```python
from build123d import *

# Parameters (mm, degrees)
F0_W         = 40.5
F0_H         = 40.5
F2_W         = 32.47
F2_H         = 32.47
F4_W         = 38
F4_H         = 38
F5_W         = 30
F5_H         = 30
F7_W         = 40.5
F7_H         = 40.5
F7_R         = 1.5
F7_R_2       = 19
F8_DEPTH     = 2.3
F9_T3_DEPTH  = 22.3515662211
F9_T6_DEPTH  = 9.05
F9_T9_DEPTH  = 9.05
F9_T12_DEPTH = 22.3515662211
F9_T15_DEPTH = 22.3515662211
F9_T18_DEPTH = 9.05
F9_T21_DEPTH = 22.3515662211
F9_T24_DEPTH = 9.05
F9_T27_DEPTH = 36.3076821333


# Not quite as in the source:
# - a fillet or chamfer that OpenCascade refuses, or shapes differently, is made with other operations: its cross-section is extruded or revolved along the edge and cut away or added


with BuildPart() as f3:
    # F0 (on Top) → F3 section 0
    with BuildSketch(Plane.XY):
        Rectangle(F0_W, F0_H)
    # F2 (on offset) → F3 section 1
    with BuildSketch(Plane.XY.offset(15)):
        Rectangle(F2_W, F2_H)
    loft()

    # F4 (on face) → F6 section 0
    with BuildSketch(Plane.XY):
        Rectangle(F4_W, F4_H)
    # F5 (on face) → F6 section 1
    with BuildSketch(Plane.XY.offset(15)):
        Rectangle(F5_W, F5_H)
    loft(mode=Mode.SUBTRACT)

    # F7 (on face) → F8 (join)
    with BuildSketch(Plane.XY):
        Rectangle(F7_W, F7_H)
        with Locations((-15.9099025767, -15.9099025767)):
            Circle(F7_R, mode=Mode.SUBTRACT)
        with Locations((15.9099025767, -15.9099025767)):
            Circle(F7_R, mode=Mode.SUBTRACT)
        with Locations((-15.9099025767, 15.9099025767)):
            Circle(F7_R, mode=Mode.SUBTRACT)
        Circle(F7_R_2, mode=Mode.SUBTRACT)
        with Locations((15.9099025767, 15.9099025767)):
            Circle(F7_R, mode=Mode.SUBTRACT)
    extrude(amount=-F8_DEPTH)

    # F9: fillet of radius 1 on 9 edges, made by hand


with BuildPart() as f9_tool1:
    # F9_s2 → F9_t3 (new body)
    with BuildSketch(Plane(origin=(-3.5329799901, -3.5329799901, -13.1991780453), x_dir=(-0.7071067812, 0.7071067812, 0), z_dir=(0.2503317407, 0.2503317407, 0.9352368893))):
        with BuildLine():
            ThreePointArc((-0.6830609237, 26.1443262584), (0, 26.4139648585), (0.6830609237, 26.1443262584))
            Line((0.6830609237, 26.1443262584), (0, 26.783150032))
            Line((0, 26.783150032), (-0.6830609237, 26.1443262584))
        make_face()
    extrude(amount=F9_T3_DEPTH)


with BuildPart() as f9_tool4:
    # F9_s5 → F9_t6 (new body)
    with BuildSketch(Plane.XY.offset(4.25)):
        with BuildLine():
            ThreePointArc((-19.25, -20.25), (-19.9571067812, -19.9571067812), (-20.25, -19.25))
            Line((-20.25, -19.25), (-20.25, -20.25))
            Line((-20.25, -20.25), (-19.25, -20.25))
        make_face()
    extrude(amount=-F9_T6_DEPTH)


with BuildPart() as f9_tool7:
    # F9_s8 → F9_t9 (new body)
    with BuildSketch(Plane.XY.offset(4.25)):
        with BuildLine():
            ThreePointArc((-20.25, 19.25), (-19.9571067812, 19.9571067812), (-19.25, 20.25))
            Line((-19.25, 20.25), (-20.25, 20.25))
            Line((-20.25, 20.25), (-20.25, 19.25))
        make_face()
    extrude(amount=-F9_T9_DEPTH)


with BuildPart() as f9_tool10:
    # F9_s11 → F9_t12 (new body)
    with BuildSketch(Plane(origin=(-3.5329799901, 3.5329799901, -13.1991780453), x_dir=(0.7071067812, 0.7071067812, 0), z_dir=(0.2503317407, -0.2503317407, 0.9352368893))):
        with BuildLine():
            ThreePointArc((-0.6830609237, 26.1443262584), (0, 26.4139648585), (0.6830609237, 26.1443262584))
            Line((0.6830609237, 26.1443262584), (0, 26.783150032))
            Line((0, 26.783150032), (-0.6830609237, 26.1443262584))
        make_face()
    extrude(amount=F9_T12_DEPTH)


with BuildPart() as f9_tool13:
    # F9_s14 → F9_t15 (new body)
    with BuildSketch(Plane(origin=(3.5329799901, 3.5329799901, -13.1991780453), x_dir=(0.7071067812, -0.7071067812, 0), z_dir=(-0.2503317407, -0.2503317407, 0.9352368893))):
        with BuildLine():
            ThreePointArc((0.6830609237, 26.1443262584), (0, 26.4139648585), (-0.6830609237, 26.1443262584))
            Line((-0.6830609237, 26.1443262584), (0, 26.783150032))
            Line((0, 26.783150032), (0.6830609237, 26.1443262584))
        make_face()
    extrude(amount=F9_T15_DEPTH)


with BuildPart() as f9_tool16:
    # F9_s17 → F9_t18 (new body)
    with BuildSketch(Plane.XY.offset(4.25)):
        with BuildLine():
            ThreePointArc((20.25, 19.25), (19.9571067812, 19.9571067812), (19.25, 20.25))
            Line((19.25, 20.25), (20.25, 20.25))
            Line((20.25, 20.25), (20.25, 19.25))
        make_face()
    extrude(amount=-F9_T18_DEPTH)


with BuildPart() as f9_tool19:
    # F9_s20 → F9_t21 (new body)
    with BuildSketch(Plane(origin=(3.5329799901, -3.5329799901, -13.1991780453), x_dir=(-0.7071067812, -0.7071067812, 0), z_dir=(-0.2503317407, 0.2503317407, 0.9352368893))):
        with BuildLine():
            ThreePointArc((0.6830609237, 26.1443262584), (0, 26.4139648585), (-0.6830609237, 26.1443262584))
            Line((-0.6830609237, 26.1443262584), (0, 26.783150032))
            Line((0, 26.783150032), (0.6830609237, 26.1443262584))
        make_face()
    extrude(amount=F9_T21_DEPTH)


with BuildPart() as f9_tool22:
    # F9_s23 → F9_t24 (new body)
    with BuildSketch(Plane.XY.offset(4.25)):
        with BuildLine():
            ThreePointArc((19.25, -20.25), (19.9571067812, -19.9571067812), (20.25, -19.25))
            Line((20.25, -19.25), (20.25, -20.25))
            Line((20.25, -20.25), (19.25, -20.25))
        make_face()
    extrude(amount=-F9_T24_DEPTH)


with BuildPart() as f9_tool25:
    # F9_s26 → F9_t27 (new body)
    with BuildSketch(Plane.XZ.offset(-18.1538410667)):
        with BuildLine():
            ThreePointArc((-15.4674635733, 15), (-16.0763295685, 14.7932730929), (-16.4334575956, 14.2585644))
            Line((-16.4334575956, 14.2585644), (-16.235, 15))
            Line((-16.235, 15), (-15.4674635733, 15))
        make_face()
    extrude(amount=F9_T27_DEPTH)


with BuildPart() as f3_1:
    add(f3.part)

    # F9_t28: cut F9_tool1, F9_tool4, F9_tool7, F9_tool10, F9_tool13, F9_tool16, F9_tool19, F9_tool22, F9_tool25
    add([f9_tool1.part, f9_tool4.part, f9_tool7.part, f9_tool10.part, f9_tool13.part, f9_tool16.part, f9_tool19.part, f9_tool22.part, f9_tool25.part], mode=Mode.SUBTRACT)


solid = f3_1.part
```
Here's how the part is built. I have some questions about the finished solid (model axes, mm). A direction names the side the tool comes from. Round coordinates to 2 decimals unless told otherwise and drop trailing zeros. Use CSV: the item, a comma, the result in double quotes.
1) I'm going to push flat-ended pins straight in: P1, Ø5, axis at y = 15, z = 10.5, coming from the -X side; P2, Ø5, axis at x = 11.5, z = 6.5, coming from the +Y side; P3, Ø1, axis at x = -2, z = 12.5, coming from the +Y side. Where does each tip first touch, or does it pass through?
Taken from the geometry:
P1,"x = -18.11"
P2,"y = 19.18"
P3,"y = 17.04"
2) If we mould it in two halves opening along Z, with no side actions, what happens to faces 4 (the cylindrical face through (-17.96, -17.98, 7.47)), 5 (the flat face through (-14, 14, 0)), 6 (the cylindrical face through (14.72, -16.82, -1.13))? For each: pulls with the +Z half, pulls with the -Z half, needs draft (parallel to the pull), parting line crosses it, or undercut.
Taken from the geometry:
face 4,"pulls with the +Z half"
face 5,"undercut"
face 6,"needs draft"
3) On a 3-axis mill with a long thin cutter (end or side, diameter ignored), from which of +Z, -Z, +X, -X, +Y, -Y can I reach the whole of each face in a straight line? I mean faces 1 (the flat face through (14, 14, 0)), 2 (the cylindrical face through (19.949, -19.965, -1.108)), 3 (the cylindrical face through (-17.02, 16.92, -1.13)). Say none if no direction works.
Taken from the geometry:
face 1,"none"
face 2,"+Z, -Z, +X, -Y"
face 3,"-Z"
4) I need wall thicknesses on line 1 along Y through (x, z) = (0, -1.75); line 2 along X through (y, z) = (-8, 3.5); line 3 along X through (y, z) = (-16, 6). Which ranges of each line are inside material? Lowest first, please. Write a range as [from, to].
Taken from the geometry:
line 1,"[-20.25, -19], [19, 20.25]"
line 2,"[-19.31, -18.07], [18.07, 19.31]"
line 3,"[-18.64, -17.4], [17.4, 18.64]"
